For this review, use the dimensioned drawing (mm, ordinates from the lowest corner) and the shaded views. Round coordinates to 2 decimals unless told otherwise and drop trailing zeros. Write each loop counter-clockwise with the first axis right and the second up, starting at its lowest first coordinate (ties: lowest second). Pieces come first, ordered by that corner, then holes. Notation, with made-up numbers: M -4.75,22 L 39.25,22 A18 ccw 39.25,37 Z; hole C 13.5,-15 d10. An arc over 180 degrees is marked long. One line per question, with ' | ' between items. Start each with the question number.
Item 1: Add section D-D, the plane z = 190.5. State the section outline as (x, y) points.
Item 2: For L1, parallel to Z at x = 114.3, y = 7.25; L2, parallel to X at y = 8.25, z = 115.5; L3, parallel to Z at x = 128, y = 7.25, list the stretches that pass through material, from the lowest coordinate up.
Item 3: Insertion check: pin 1 Ø3 at (y, z) = (10.5, 166.5) entering from +X; pin 2 Ø5 at (x, y) = (166, 11.5) entering from +Z; pin 3 Ø2 at (x, y) = (202, 7) entering from -Z. Each pin has a flat end and moves straight along its axis. Give the tip position at first contact, or say it passes through.
Item 4: Add section B-B, the plane x = 114.3. State the section outline as (y, z) points, and give its area (3 significant figures).
Item 5: Add section A-A, the plane z = 114.3. State the section outline as (x, y) points.
Item 6: Draft analysis for pull direction Z (two halves, no side actions). For the marked faces 1, 2 and 3, state which applies: released by +Z, released by -Z, zero draft, split by the parting line, or undercut.
Item 7: Add section C-C, the plane y = 6.5. State the section outline as (x, z) points, and give its area (3 significant figures).
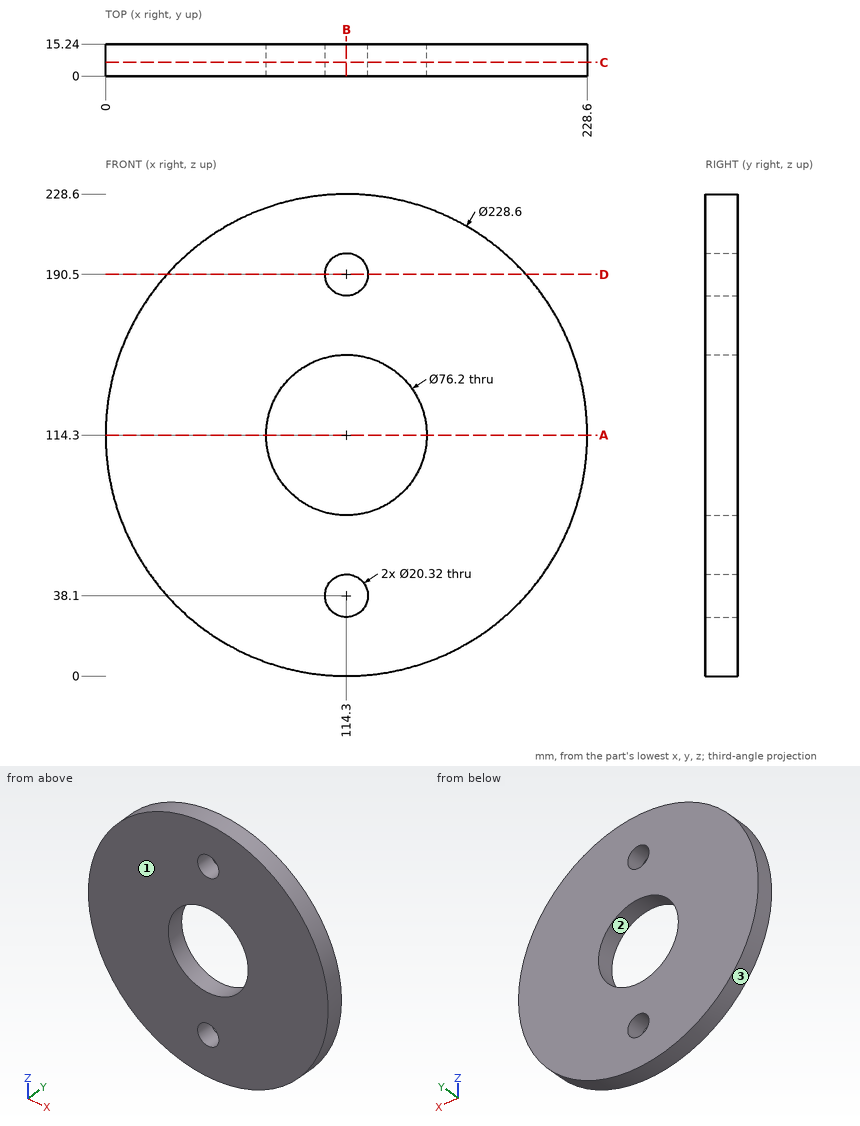
Computed values:
1) outline: M 29.11,0 L 104.14,0 L 104.14,15.24 L 29.11,15.24 Z; M 124.46,0 L 199.49,0 L 199.49,15.24 L 124.46,15.24 Z
2) L1: z = 0 to 27.94, 48.26 to 76.2, 152.4 to 180.34, 200.66 to 228.6 | L2: x = 0.01 to 76.22, 152.38 to 228.59 | L3: z = 0.82 to 78.75, 149.85 to 227.78
3) pin 1: stops at x = 216.74 | pin 2: stops at z = 217.47 | pin 3: stops at z = 39.82
4) outline: M 0,0 L 15.24,0 L 15.24,27.94 L 0,27.94 Z; M 0,48.26 L 15.24,48.26 L 15.24,76.2 L 0,76.2 Z; M 0,152.4 L 15.24,152.4 L 15.24,180.34 L 0,180.34 Z; M 0,200.66 L 15.24,200.66 L 15.24,228.6 L 0,228.6 Z | area: 1,700 mm^2
5) outline: M 0,0 L 76.2,0 L 76.2,15.24 L 0,15.24 Z; M 152.4,0 L 228.6,0 L 228.6,15.24 L 152.4,15.24 Z
6) face 1: zero draft | face 2: undercut | face 3: split by the parting line
7) outline: C 114.3,114.3 d228.6; hole C 114.3,114.3 d76.2; hole C 114.3,38.1 d20.32; hole C 114.3,190.5 d20.32 | area: 35,800 mm^2
